Geometry: final body of the model. Coordinates: model frame, mm. Give positions to 0.01 mm unless a question says otherwise; leave off trailing zeros. One line per item, written item: value. Start each with the question number.
```python
from build123d import *

# Parameters (mm, degrees)
CUT_EXTRUDE1_REACH             = 53.79
SKETCH5_R                      = 3
CUT_EXTRUDE1_DIRECTION_2_REACH = 53.79
CUT_EXTRUDE2_DEPTH             = 52.790443273
FILLET1_R                      = 2
CIRPATTERN2_COUNT              = 12
FILLET1_OF_CIRPATTERN2_R       = 2


with BuildPart() as part:
    # Sketch3 → Revolve1 (revolve)
    with BuildSketch(Plane.XY, mode=Mode.PRIVATE) as revolve1_sk:
        with BuildLine():
            Line((9.5, 0), (9.5, 26.5))
            ThreePointArc((9.5, 26.5), (0, 36), (-9.5, 26.5))
            Line((-9.5, 26.5), (-9.5, 0))
            Line((-9.5, 0), (9.5, 0))
        make_face()
    revolve(revolve1_sk.sketch.rotate(Axis((-15.081723319, 0, 0), (1, 0, 0)), 90), axis=Axis((-15.081723319, 0, 0), (1, 0, 0)))

    # Sketch5 → Cut-Extrude1 (cut, up to next)
    with BuildSketch(Plane(origin=(0, 0, 0), x_dir=(0, 0, -1), z_dir=(1, 0, 0)), mode=Mode.PRIVATE) as cut_extrude1_sk1:
        with Locations(Location((0, 0, 0), (0, 0, 180))):
            Circle(SKETCH5_R)
    cut_extrude1_tool1 = extrude(cut_extrude1_sk1.sketch, amount=-CUT_EXTRUDE1_REACH, mode=Mode.PRIVATE) & part.part
    add(cut_extrude1_tool1.solids().sort_by_distance((0, 0, 0))[0], mode=Mode.SUBTRACT)

    # Sketch5 → Cut-Extrude1 direction 2 (cut, up to next)
    with BuildSketch(Plane(origin=(0, 0, 0), x_dir=(0, 0, -1), z_dir=(1, 0, 0)), mode=Mode.PRIVATE) as cut_extrude1_direction_2_sk1:
        with Locations(Location((0, 0, 0), (0, 0, 180))):
            Circle(SKETCH5_R)
    cut_extrude1_direction_2_tool1 = extrude(cut_extrude1_direction_2_sk1.sketch, amount=CUT_EXTRUDE1_DIRECTION_2_REACH, mode=Mode.PRIVATE) & part.part
    add(cut_extrude1_direction_2_tool1.solids().sort_by_distance((0, 0, 0))[0], mode=Mode.SUBTRACT)

    # Sketch6 → Cut-Extrude2 (cut, symmetric)
    with BuildSketch(Plane(origin=(0, 0, 0), x_dir=(0, 0, -1), z_dir=(1, 0, 0))):
        with BuildLine():
            Line((-3.646611731, 20.680962813), (-2.25742631, 12.802500789))
            ThreePointArc((-2.25742631, 12.802500789), (0, 13), (2.25742631, 12.802500789))
            Line((2.25742631, 12.802500789), (3.646611731, 20.680962813))
            ThreePointArc((3.646611731, 20.680962813), (0, 21), (-3.646611731, 20.680962813))
        make_face()
    cut_extrude2 = extrude(amount=CUT_EXTRUDE2_DEPTH, both=True, mode=Mode.SUBTRACT)

    # Fillet1
    fillet1_edges = [part.edges().sort_by_distance(p)[0] for p in [
        (0, 20.680962813, 3.646611731),
        (0, 20.680962813, -3.646611731),
        (0, 12.802500789, -2.25742631),
        (0, 12.802500789, 2.25742631),
    ]]
    fillet(fillet1_edges, radius=FILLET1_R)

    # CirPattern2: Cut-Extrude2 ×12 about axis
    cirpattern2_axis = Axis((0, 0, 0), (1, 0, 0))
    for i in range(1, CIRPATTERN2_COUNT):
        add(cut_extrude2.rotate(cirpattern2_axis, i * 360 / CIRPATTERN2_COUNT), mode=Mode.SUBTRACT)

    # Fillet1 of CirPattern2
    fillet1_of_cirpattern2_edges = [part.edges().sort_by_distance(p)[0] for p in [
        (0, 16.086933305, 13.498539803),
        (0, 19.733545037, 7.18242301),
        (0, 12.21600407, 4.446261863),
        (0, 9.958577761, 8.356238926),
        (0, 7.18242301, 19.733545037),
        (0, 13.498539803, 16.086933305),
        (0, 8.356238926, 9.958577761),
        (0, 4.446261863, 12.21600407),
        (0, -3.646611731, 20.680962813),
        (0, 3.646611731, 20.680962813),
        (0, 2.25742631, 12.802500789),
        (0, -2.25742631, 12.802500789),
        (0, -13.498539803, 16.086933305),
        (0, -7.18242301, 19.733545037),
        (0, -4.446261863, 12.21600407),
        (0, -8.356238926, 9.958577761),
        (0, -19.733545037, 7.18242301),
        (0, -16.086933305, 13.498539803),
        (0, -9.958577761, 8.356238926),
        (0, -12.21600407, 4.446261863),
        (0, -20.680962813, -3.646611731),
        (0, -20.680962813, 3.646611731),
        (0, -12.802500789, 2.25742631),
        (0, -12.802500789, -2.25742631),
        (0, -16.086933305, -13.498539803),
        (0, -19.733545037, -7.18242301),
        (0, -12.21600407, -4.446261863),
        (0, -9.958577761, -8.356238926),
        (0, -7.18242301, -19.733545037),
        (0, -13.498539803, -16.086933305),
        (0, -8.356238926, -9.958577761),
        (0, -4.446261863, -12.21600407),
        (0, 3.646611731, -20.680962813),
        (0, -3.646611731, -20.680962813),
        (0, -2.25742631, -12.802500789),
        (0, 2.25742631, -12.802500789),
        (0, 13.498539803, -16.086933305),
        (0, 7.18242301, -19.733545037),
        (0, 4.446261863, -12.21600407),
        (0, 8.356238926, -9.958577761),
        (0, 19.733545037, -7.18242301),
        (0, 16.086933305, -13.498539803),
        (0, 9.958577761, -8.356238926),
        (0, 12.21600407, -4.446261863),
    ]]
    fillet(fillet1_of_cirpattern2_edges, radius=FILLET1_OF_CIRPATTERN2_R)


solid = part.part
```
Q1. Contact query for flat-ended pins moving along their axis: pin 1 (2 mm diameter, centred on x = -0.5, y = -23.5, fed in from +Z); pin 2 (1.5 mm diameter, centred on x = -5, y = -15.5, fed in from +Z); pin 3 (10 mm diameter, centred on x = 1, y = 10.5, fed in from +Z). Output: stop coordinate, or through.
Q2. Section query A-A on x = 2.5. Give the number of separate pieces and of enclosed holes in the cut face, and give its area (3 significant figures).
Q3. Ray query, line 1 along Z through (x, y) = (7.5, 15.5); line 2 along Y through (x, z) = (-7.5, 12); line 3 along Y through (x, z) = (4.25, 0). Return the intervals inside material, ascending. Write a range as [from, to].
Q4. Mould query, pull axis Z, two halves, no side actions, for faces 1 (the face through (0.133, -1.85, -13.417)), 2 (the face through (-9.5, 6, 0)). Classes: +Z half, -Z half, draft (parallel to the pull), parting line (faces both ways), or undercut.
Results below:
1. pin 1: z = 28.09
1. pin 2: z = 31.51
1. pin 3: z = 35.57
2. separate pieces: 1
2. enclosed holes: 13
2. area: 3,440 mm2
3. line 1: [-28.37, -12.6], [-5.64, -2.73], [2.73, 5.64], [12.6, 28.37]
3. line 2: [-30.02, -17.2], [-14.3, -10.07], [-5.43, 5.43], [10.07, 14.3], [17.2, 30.02]
3. line 3: [-35, -21], [-13, -3], [3, 13], [21, 35]
4. face 1: undercut
4. face 2: draft
